```python
from build123d import *

# Parameters (mm, degrees)
SCHIZZO1_W                     = 74.3
SCHIZZO1_H                     = 20
ESTRUSIONE_ESTRUSIONE1_DEPTH   = 5
SCHIZZO2_W                     = 4
SCHIZZO2_H                     = 20
ESTRUSIONE_ESTRUSIONE2_DEPTH   = 85
ESTRUSIONE_ESTRUSIONE2_2_DEPTH = 85
SCHIZZO3_W                     = 4
SCHIZZO3_H                     = 20
ESTRUSIONE_ESTRUSIONE3_DEPTH   = 5
SCHIZZO4_W                     = 5
SCHIZZO4_H                     = 20
ESTRUSIONE_ESTRUSIONE4_DEPTH   = 12
SCHIZZO5_R                     = 1.5
TAGLIO_ESTRUSIONE1_DEPTH       = 101.746823771
SCHIZZO6_W                     = 5
SCHIZZO6_H                     = 20
ESTRUSIONE_ESTRUSIONE5_DEPTH   = 12
RACCORDO1_R                    = 4


with BuildPart() as part:
    # Schizzo1 → Estrusione-Estrusione1 (new body)
    with BuildSketch(Plane.XY):
        Rectangle(SCHIZZO1_W, SCHIZZO1_H)
    extrude(amount=ESTRUSIONE_ESTRUSIONE1_DEPTH)



with BuildPart() as body_2:
    # Schizzo2 → Estrusione-Estrusione2 (new body)
    with BuildSketch(Plane.XY.offset(5)):
        with Locations((-39.15, 0)):
            Rectangle(SCHIZZO2_W, SCHIZZO2_H)
    extrude(amount=ESTRUSIONE_ESTRUSIONE2_DEPTH)


with BuildPart() as body_3:
    # Schizzo2 → Estrusione-Estrusione2 2 (new body)
    with BuildSketch(Plane.XY.offset(5)):
        with Locations((39.15, 0)):
            Rectangle(SCHIZZO2_W, SCHIZZO2_H)
    extrude(amount=ESTRUSIONE_ESTRUSIONE2_2_DEPTH)


with BuildPart() as part_1:
    add(part.part)

    add(body_2.part)  # Estrusione-Estrusione3 merges body 2

    add(body_3.part)  # Estrusione-Estrusione3 merges body 3
    # Schizzo3 → Estrusione-Estrusione3 (add)
    with BuildSketch(Plane(origin=(0, 0, 5), x_dir=(-1, 0, 0), z_dir=(0, 0, -1))):
        with Locations((-39.15, 0)):
            Rectangle(SCHIZZO3_W, SCHIZZO3_H)
        with Locations((39.15, 0)):
            Rectangle(SCHIZZO3_W, SCHIZZO3_H)
    extrude(amount=ESTRUSIONE_ESTRUSIONE3_DEPTH)

    # Schizzo4 → Estrusione-Estrusione4 (add)
    with BuildSketch(Plane(origin=(41.15, 0, 0), x_dir=(0, 0, -1), z_dir=(1, 0, 0))):
        with Locations((-87.5, 0)):
            Rectangle(SCHIZZO4_W, SCHIZZO4_H)
    extrude(amount=ESTRUSIONE_ESTRUSIONE4_DEPTH)

    # Schizzo5 → Taglio-Estrusione1 (cut, through all)
    with BuildSketch(Plane(origin=(0, 0, 85), x_dir=(-1, 0, 0), z_dir=(0, 0, -1))):
        with Locations((-47.15, 0)):
            Circle(SCHIZZO5_R)
    taglio_estrusione1 = extrude(amount=-TAGLIO_ESTRUSIONE1_DEPTH, mode=Mode.SUBTRACT)

    # Schizzo6 → Estrusione-Estrusione5 (add)
    with BuildSketch(Plane.ZY.offset(41.15)):
        with Locations((87.5, 0)):
            Rectangle(SCHIZZO6_W, SCHIZZO6_H)
    extrude(amount=ESTRUSIONE_ESTRUSIONE5_DEPTH)

    # Specchia13: Taglio-Estrusione1 across plane
    add(taglio_estrusione1.mirror(Plane(origin=(0, 0, 0), x_dir=(0, 0, 1), z_dir=(1, 0, 0))), mode=Mode.SUBTRACT)

    # Raccordo1
    raccordo1_edges = [part_1.edges().sort_by_distance(p)[0] for p in [
        (-41.15, 0, 85),
        (-53.15, 10, 87.5),
        (-53.15, -10, 87.5),
        (41.15, 0, 0),
        (-41.15, 0, 0),
        (41.15, 0, 85),
        (53.15, -10, 87.5),
        (53.15, 10, 87.5),
    ]]
    fillet(raccordo1_edges, radius=RACCORDO1_R)


solid = part_1.part
```
Work out the finished part from the listing and answer in its coordinate system (mm). A direction names the side the tool comes from. Give positions to 0.01 mm unless a question says otherwise; leave off trailing zeros. Loops run counter-clockwise (first coordinate to the right, second up) from the corner with the lowest first, then second, coordinate; pieces in that order, holes last. Notation, with made-up numbers: M -35.5,45.5 L 12.5,45.5 A9 cw 12.5,60.5 Z; hole C 19,-32 d8. An arc over 180 degrees is marked long. One line per item, written item: value. Start each with the question number.
1. Find section B-B (x = 47.15). Give the vertices of the cut face in (y, z), and give its area (3 significant figures).
2. Find section C-C (y = 0). Give the vertices of the cut face in (x, z), and give its area (3 significant figures).
3. Find section A-A (z = 41). Give the vertices of the cut face in (x, y).
4. Find section D-D (x = -35). Give the vertices of the cut face in (y, z), and give its area (3 significant figures).
5. Determine the mould class of faces 1 (the face through (40.009, 0.14, 1.203)), 2 (the face through (0.2, -10, 4.8)), 3 (the face through (37.15, 0, 47)) for opening direction X: released by +X, released by -X, zero draft, split by the parting line, or undercut.
6. Each of these flat-tipped pins is pushed along its axis until it touches: P1, Ø2, axis at y = -0.5, z = 22.5, coming from the +X side; P2, Ø8, axis at x = -29.5, y = -7.5, coming from the +Z side; P3, Ø8, axis at y = -0.5, z = 42, coming from the -X side. Where does it stop, or does it pass through?
7. Find the intervals of material crossed by probe 1 along Y at (x, z) = (47.15, 87.3); probe 2 along X at (y, z) = (5.25, 44); probe 3 along Z at (x, y) = (35, 4), in increasing order.
8. Which of the six approach directions +Z, -Z, +X, -X, +Y, -Y give full straight-line access (tool end or side, diameter ignored) to faces 4 (the face through (49, 0, 85)), 5 (the face through (-49, 0, 85)), 6 (the face through (-37.15, 0, 47))?
Reported:
1. outline: M -10,85 L -1.5,85 L -1.5,90 L -10,90 Z; M 1.5,85 L 10,85 L 10,90 L 1.5,90 Z
1. area: 85.0 mm²
2. outline: M -53.15,85 L -48.65,85 L -48.65,90 L -53.15,90 Z; M -45.65,85 L -45.15,85 A4 cw -41.15,81 L -41.15,4 A4 ccw -37.15,0 L 37.15,0 A4 ccw 41.15,4 L 41.15,81 A4 cw 45.15,85 L 45.65,85 L 45.65,90 L 37.15,90 L 37.15,5 L -37.15,5 L -37.15,90 L -45.65,90 Z; M 48.65,85 L 53.15,85 L 53.15,90 L 48.65,90 Z
2. area: 1,180 mm²
3. outline: M -41.15,-10 L -37.15,-10 L -37.15,10 L -41.15,10 Z; M 37.15,-10 L 41.15,-10 L 41.15,10 L 37.15,10 Z
4. outline: M -10,0 L 10,0 L 10,5 L -10,5 Z
4. area: 100 mm²
5. face 1: released by +X
5. face 2: zero draft
5. face 3: undercut
6. P1: stops at x = 41.15
6. P2: stops at z = 5
6. P3: stops at x = -41.15
7. probe 1: y = -10 to -1.5, 1.5 to 10
7. probe 2: x = -41.15 to -37.15, 37.15 to 41.15
7. probe 3: z = 0 to 5
8. face 4: -Z, +X, +Y, -Y
8. face 5: -Z, -X, +Y, -Y
8. face 6: +Z, +Y, -Y
